Here's how the part is built. I have some questions about the finished solid (model axes, mm). Face numbers are marked on the shaded views. Round coordinates to 2 decimals unless told otherwise and drop trailing zeros. Write each loop counter-clockwise with the first axis right and the second up, starting at its lowest first coordinate (ties: lowest second). Pieces come first, ordered by that corner, then holes. Notation, with made-up numbers: (-14, 27.25) -> (13, 27.25) arc R19 ccw to (13, 48.25) -> close; hole circle Ø6 at (-22.5, -10.5). An arc over 180 degrees is marked (long way). Answer in a Markdown table with one row per item. Add a question column.
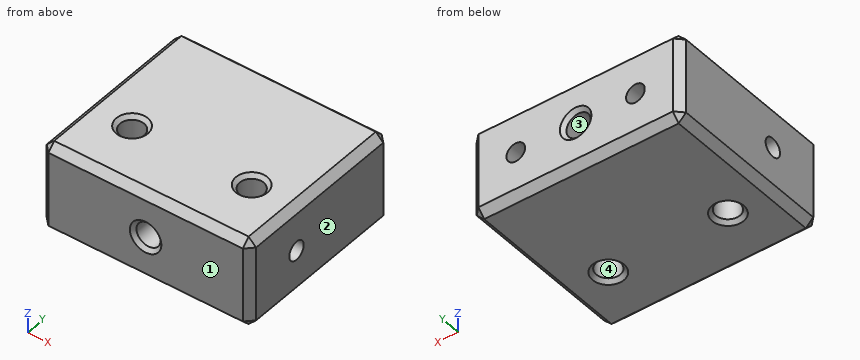
Autodesk Inventor part; units mm, degrees
ref_plane "Work Plane1" through (0, -25.4, 0) normal (0, 1, 0) x (-1, 0, 0)
ref_plane "YZ Plane" through (0, 0, 0) normal (1, 0, 0) x (0, 1, 0)
ref_plane "XY Plane" through (0, 0, 0) normal (0, 0, 1) x (1, 0, 0)
sketch "Sketch2" plane through (0, 0, 0) normal (0, 1, 0) x (-1, 0, 0)
  line L0 (0, -13.335) -> (0, 13.335) construction
  line L1 (-31.115, 0) -> (31.115, 0) construction
  line L2 (22.225, 9.525) -> (-22.225, 9.525)
  line L3 (-22.225, 9.525) -> (-22.225, -9.525)
  line L4 (-22.225, -9.525) -> (22.225, -9.525)
  line L5 (22.225, -9.525) -> (22.225, 9.525)
  point P0 (0, 0)
  point P1 (0, 0)
  point P2 (-12.7, 0)
  point P3 (12.7, 0)
  dimension "d0" = 19.05
  dimension "d1" = 44.45
  dimension "d5" = 25.4
extrude "Extrusion1" add sketch "Sketch2" against normal blind 38.1
hole "Hole1" at (0, 0, 0) direction (0, -1, 0) diameter 5.1054 end through all
hole "Hole2" at (12.7, 0, 0) at (-12.7, 0, 0) direction (0, -1, 0) diameter 3.9624 depth 13.6144 tip angle 118
ref_plane "Work Plane1" through (0, -25.4, 0) normal (0, 1, 0) x (-1, 0, 0)
sketch "Sketch3" plane through (22.225, 0, -9.525) normal (0, 0, -1) x (-1, 0, 0)
  line L0 (22.225, -45.72) -> (22.225, 7.62) construction
  line L1 (-8.89, -25.4) -> (53.34, -25.4) construction
  line L2 (-8.89, 0) -> (53.34, 0) construction
  point P0 (22.225, 0)
  point P1 (34.925, -25.4)
  point P2 (9.525, -25.4)
  dimension "d21" = 25.4
hole "Hole3" at (-12.7, -25.4, -9.525) at (12.7, -25.4, -9.525) direction (0, 0, 1) diameter 5.1054 end through all
sketch "Sketch4" plane through (0, -25.4, 0) normal (0, 1, 0) x (-1, 0, 0)
  point P0 (0, 0)
sketch "Sketch5" plane through (-22.225, 0, -9.525) normal (-1, 0, 0) x (0, 0, 1)
  line L0 (9.525, 7.62) -> (9.525, -45.72) construction
  line L1 (-3.81, 0) -> (22.86, 0) construction
  line L2 (-3.81, -25.4) -> (22.86, -25.4) construction
  point P0 (9.525, 0)
  point P1 (9.525, -25.4)
hole "Hole4" at (-22.225, -25.4, 0) direction (1, 0, 0) diameter 3.9624 depth 13.6144 tip angle 118
mirror "Mirror1" about plane through (0, 0, 0) normal (1, 0, 0) of "Hole4"
chamfer "Chamfer1" distance 1.5875 angle 45 12 edges at (-22.225, -19.05, -9.525) (22.225, -19.05, -9.525) (-22.225, -19.05, 9.525) (22.225, -19.05, 9.525) (0, 0, 9.525) (0, 0, -9.525) (-22.225, 0, 0) (22.225, 0, 0) (0, -38.1, 9.525) (22.225, -38.1, 0) (0, -38.1, -9.525) (-22.225, -38.1, 0)
chamfer "Chamfer2" distance 0.7937 angle 45 6 edges at (-12.7, -27.9527, 9.525) (12.7, -27.9527, 9.525) (12.7, -27.9527, -9.525) (-12.7, -27.9527, -9.525) (0, 0, -2.5527) (0, -38.1, -2.5527)
properties part number "5190-16-0001" material "Aluminum 6061"
Item 1: For P1, Ø2.5, axis at y = -25.4, z = 0, coming from the -X side; P2, Ø3, axis at y = -25.4, z = 0, coming from the +X side; P3, Ø3, axis at x = -12.7, z = 0, coming from the +Y side, each with a flat end and sliding along its axis, tell me the tip position at first contact or that it passes through.
Item 2: If we mould it in two halves opening along X, with no side actions, what happens to the marked faces 1, 2, 3 and 4? For each: pulls with the +X half, pulls with the -X half, needs draft (parallel to the pull), parting line crosses it, or undercut.
Item 3: If we section it at B-B on y = -31: Please give me the cut outline in (x, z) (1 decimal).
Item 4: I need wall thicknesses on line 1 along X through (y, z) = (-13, 0) (3 decimals); line 2 along X through (y, z) = (-25.4, 2.75) (3 decimals); line 3 along Y through (x, z) = (9.2, 0). Which ranges of each line are inside material? Lowest first, please. Write a range as from..to.
Item 5: If we section it at D-D on y = -10: Please give me the cut outline in (x, z) (1 decimal).
Item 6: If we section it at C-C on x = -17.5: Please give me the cut outline in (y, z) (1 decimal).
Item 7: If we section it at A-A on z = 6.5: Please give me the cut outline in (x, y) (1 decimal).
Results list:
| question | item | result |
|---|---|---|
| 1 | P1 | x = -8.17 |
| 1 | P2 | x = 8.32 |
| 1 | P3 | y = -13.9 |
| 2 | face 1 | needs draft |
| 2 | face 2 | pulls with the +X half |
| 2 | face 3 | undercut |
| 2 | face 4 | undercut |
| 3 | outline | (-22.2, -7.9) -> (-20.6, -9.5) -> (20.6, -9.5) -> (22.2, -7.9) -> (22.2, 7.9) -> (20.6, 9.5) -> (-20.6, 9.5) -> (-22.2, 7.9) -> close; hole circle Ø5.1 at (0, 0) |
| 4 | line 1 | -22.225..-14.681, -10.719..-2.553, 2.553..10.719, 14.681..22.225 |
| 4 | line 2 | -22.225..-15.253, -10.147..10.147, 15.253..22.225 |
| 4 | line 3 | -38.1..-27.38, -23.42..0 |
| 5 | outline | (-22.2, -7.9) -> (-20.6, -9.5) -> (20.6, -9.5) -> (22.2, -7.9) -> (22.2, 7.9) -> (20.6, 9.5) -> (-20.6, 9.5) -> (-22.2, 7.9) -> close; hole circle Ø4 at (-12.7, 0); hole circle Ø5.1 at (0, 0); hole circle Ø4 at (12.7, 0) |
| 6 | outline | (-38.1, -7.9) -> (-36.5, -9.5) -> (-1.6, -9.5) -> (0, -7.9) -> (0, 7.9) -> (-1.6, 9.5) -> (-36.5, 9.5) -> (-38.1, 7.9) -> close; hole circle Ø4 at (-25.4, 0) |
| 7 | outline | (-22.2, -36.5) -> (-20.6, -38.1) -> (20.6, -38.1) -> (22.2, -36.5) -> (22.2, -1.6) -> (20.6, 0) -> (-20.6, 0) -> (-22.2, -1.6) -> close; hole circle Ø5.1 at (-12.7, -25.4); hole circle Ø5.1 at (12.7, -25.4) |
